Here's how the part is built. I have some questions about the finished solid (model axes, mm). A direction names the side the tool comes from. Give positions to 0.01 mm unless a question says otherwise; leave off trailing zeros. Order: outer loops, then holes, each group sorted by start corner. A loop starts at its lowest first (then second) coordinate and runs counter-clockwise, first axis right, second up. Notation, with made-up numbers: (71.5, -0.5) - (79.5, -0.5) arc R12 ccw to (79.5, 22.5) - close; hole circle Ø8 at (-32, 50.5). An arc over 180 degrees is marked (long way). One line per question, with ' | ' between items.
from build123d import *

# Parameters (mm, degrees)
BOSS_EXTRUDE1_DEPTH = 10
BOSS_EXTRUDE2_DEPTH = 22
SKETCH3_R           = 6
CUT_EXTRUDE1_DEPTH  = 24
LPATTERN1_COUNT     = 2
LPATTERN1_PITCH     = 16
FILLET1_R           = 3
FILLET2_R           = 3


# Read off the part's stored shape, not the designer's step: CBORE for M5 Hex Head Bolt1
with BuildPart() as part:
    # Sketch1 → Boss-Extrude1 (new body)
    with BuildSketch(Plane(origin=(0, 0, 0), x_dir=(0, 0, -1), z_dir=(1, 0, 0))):
        Polygon((-32, 45), (32, 45), (32, 9), (8, 9), (8, 0), (-8, 0), (-8, 9), (-32, 9), align=None)
    extrude(amount=BOSS_EXTRUDE1_DEPTH)

    # Sketch2 → Boss-Extrude2 (add)
    with BuildSketch(Plane(origin=(10, 0, 0), x_dir=(0, 0, -1), z_dir=(1, 0, 0))):
        with BuildLine():
            Line((0, 45), (0, 0))
            Line((0, 0), (8, 0))
            Line((8, 0), (8, 9))
            Line((8, 9), (32, 9))
            Line((32, 9), (32, 19))
            Line((32, 19), (27.5, 19))
            Line((27.5, 19), (12.8, 38.6))
            ThreePointArc((12.8, 38.6), (7.155417528, 43.310835056), (0, 45))
        make_face()
        with BuildLine():
            Line((-32, 9), (-8, 9))
            Line((-8, 9), (-8, 0))
            Line((-8, 0), (0, 0))
            Line((0, 0), (0, 45))
            ThreePointArc((0, 45), (-7.155417528, 43.310835056), (-12.8, 38.6))
            Line((-12.8, 38.6), (-27.5, 19))
            Line((-27.5, 19), (-32, 19))
            Line((-32, 19), (-32, 9))
        make_face()
    extrude(amount=BOSS_EXTRUDE2_DEPTH)

    # Sketch3 → Cut-Extrude1 (cut)
    with BuildSketch(Plane(origin=(32, 0, 0), x_dir=(0, 0, -1), z_dir=(1, 0, 0))):
        with Locations((0, 29)):
            Circle(SKETCH3_R)
    extrude(amount=-CUT_EXTRUDE1_DEPTH, mode=Mode.SUBTRACT)

    # CBORE for M5 Hex Head Bolt1 outline → CBORE for M5 Hex Head Bolt1 (revolve, cut)
    with BuildSketch(Plane(origin=(20, 0, 0), x_dir=(1, 0, 0), z_dir=(0, 0, 1))):
        Polygon((0, 34.195854076), (3, 34.195854076), (3, 41), (5, 41), (5, 45.000103319), (0, 45.000103319), align=None)
    revolve(axis=Axis((20, 0, 0), (0, 1, 0)), mode=Mode.SUBTRACT)

    # Sketch7 → Tap Drill for M2.2 Helicoil1 (revolve, cut)
    with BuildSketch(Plane(origin=(24, 0, 0), x_dir=(0, 0, -1), z_dir=(1, 0, 0))):
        Polygon((0, 0), (0, 16.66395281), (1.15, 16), (1.15, 0), align=None)
    tap_drill_for_m2_2_helicoil1 = revolve(axis=Axis((24, -6.35, 0), (0, 1, 0)), mode=Mode.SUBTRACT)

    # LPattern1: Tap Drill for M2.2 Helicoil1 ×2
    with Locations(*[(-i * LPATTERN1_PITCH, 0, 0) for i in range(1, LPATTERN1_COUNT)]):
        add(tap_drill_for_m2_2_helicoil1, mode=Mode.SUBTRACT)

    # Fillet1
    fillet1_edges = [part.edges().sort_by_distance(p)[0] for p in [
        (21, 19, 27.5),
    ]]
    fillet(fillet1_edges, radius=FILLET1_R)

    # Fillet2
    fillet2_edges = [part.edges().sort_by_distance(p)[0] for p in [
        (21, 19, -27.5),
    ]]
    fillet(fillet2_edges, radius=FILLET2_R)


solid = part.part
1) I want a section at C-C (z = 10). List the corners of the cut face in (x, y) for me, plus the area to 3 significant figures.
Model answer:
outline: (0, 9) - (32, 9) - (32, 41.49) - (10, 41.49) - (10, 45) - (0, 45) - close | area: 1,070 mm2
2) I want a section at B-B (y = 37). List the corners of the cut face in (x, z) for me, plus the area to 3 significant figures.
Model answer:
outline: (0, -32) - (10, -32) - (10, -14) - (32, -14) - (32, 14) - (10, 14) - (10, 32) - (0, 32) - close; hole circle Ø6 at (20, 0) | area: 1,230 mm2
3) On a 3-axis mill with a long thin cutter (end or side, diameter ignored), from which of +Z, -Z, +X, -X, +Y, -Y can I reach the whole of each face in a straight line? I mean faces 5 (the face through (25.123, 7.888, 0.249)), 6 (the face through (21.154, 19.308, 27.676)), 7 (the face through (26, 45, 0)), 8 (the face through (21, 19, -31)), 9 (the face through (16, 5, 8)). Say none if no direction works.
Model answer:
face 5: -Y | face 6: +Z, +X, +Y | face 7: +X, +Y | face 8: -Z, +X, +Y | face 9: +Z, +X, -X, -Y
4) Please list where these lines run through material, in increasing order: L1, parallel to X at y = 4, z = 0; L2, parallel to Z at x = 8, y = 7.25; L3, parallel to Y at x = 28.5, z = 29.5.
Model answer:
L1: x = 0 to 6.85, 9.15 to 22.85, 25.15 to 32 | L2: z = -8 to -1.15, 1.15 to 8 | L3: y = 9 to 19
5) Thinking about a two-plate mould opening in Y: for faces 1 (the face through (21.154, 19.325, -27.641)), 2 (the face through (20.168, 23.143, 1.301)), 3 (the face through (10, 35, -23)), 4 (the face through (8, 29, 0)), which applies, +Y half, -Y half, draft (parallel to the pull), parting line (faces both ways), or undercut?
Model answer:
face 1: +Y half | face 2: undercut | face 3: draft | face 4: undercut
6) I want a section at D-D (y = 29). List the corners of the cut face in (x, z) for me, plus the area to 3 significant figures.
Model answer:
outline: (0, -32) - (10, -32) - (10, -20) - (32, -20) - (32, -6) - (8, -6) - (8, 6) - (32, 6) - (32, 20) - (10, 20) - (10, 32) - (0, 32) - close | area: 1,230 mm2
7) I want a section at A-A (x = 28). List the corners of the cut face in (y, z) for me, plus the area to 3 significant figures.
Model answer:
outline: (0, -8) - (9, -8) - (9, -32) - (19, -32) - (19, -29) arc R3 cw to (20.2, -26.6) - (38.6, -12.8) arc R16 ccw to (38.6, 12.8) - (20.2, 26.6) arc R3 cw to (19, 29) - (19, 32) - (9, 32) - (9, 8) - (0, 8) - close; hole circle Ø12 at (29, 0) | area: 1,580 mm2
8) I'm going to push flat-ended pins straight in: P1, Ø0.9, axis at x = 17.5, z = 31, coming from the +Y side; P2, Ø2.5, axis at x = 11.5, y = 6.5, coming from the -Z side; P3, Ø5, axis at x = 20, z = 0, coming from the +Y side. Where does each tip first touch, or does it pass through?
Model answer:
P1: stops at y = 19 | P2: stops at z = -8 | P3: stops at y = 23.55
